```python
from build123d import *

# Parameters (mm, degrees)
F1_DEPTH = 25


with BuildPart() as f1:
    # F0 (on Top) → F1 (new body)
    with BuildSketch(Plane.XY):
        Polygon((0, 40), (-38.992442, 0), (-35.412103, -3.490154), (-12.513641, 20), (0, 32.836992), (13.168698, 20), (37.265833, -3.490154), (41.033594, 0), align=None)
        Polygon((0, 32.836992), (-12.513641, 20), (13.168698, 20), align=None)
    extrude(amount=F1_DEPTH)


solid = f1.part
```
Work out the finished part from the listing and answer in its coordinate system (mm). A direction names the side the tool comes from. Coordinates: 2 decimals unless noted, no trailing zeros. Loops run counter-clockwise (first coordinate to the right, second up) from the corner with the lowest first, then second, coordinate; pieces in that order, holes last.
1) Section B-B (y = 14) is taken. Give the vertices of the cut face in (x, z), plus the area to 3 significant figures.
Results:
outline: (-25.35, 0) - (-18.36, 0) - (-18.36, 25) - (-25.35, 25) - close; (19.32, 0) - (26.67, 0) - (26.67, 25) - (19.32, 25) - close
area: 358 mm2
2) Consider probe 1 along X at (y, z) = (10, 16); probe 2 along X at (y, z) = (7, 10.5); probe 3 along X at (y, z) = (20.5, 15.5). Determine where each line is inside the solid, lowest interval first.
Results:
probe 1: x = -29.24 to -22.26, 23.43 to 30.78
probe 2: x = -32.17 to -25.19, 26.5 to 33.85
probe 3: x = -19.01 to 20
3) Section C-C (x = 6) is taken. Give the vertices of the cut face in (y, z).
Results:
outline: (20, 0) - (34.15, 0) - (34.15, 25) - (20, 25) - close
4) Flat-ended cylindrical pins translate along their axes: pin 1 (8 mm diameter, centred on y = 7.5, z = 5, fed in from +X); pin 2 (3 mm diameter, centred on x = 16.5, z = 3, fed in from +Y); pin 3 (8 mm diameter, centred on x = -26, z = 19.5, fed in from -Y). Find the tip coordinate at first contact, or state that the pin passes through.
Results:
pin 1: stops at x = 37.44
pin 2: stops at y = 25.38
pin 3: stops at y = 2.06
5) Section A-A (z = 14.5) is taken. Give the vertices of the cut face in (x, y), plus the area to 3 significant figures.
Results:
outline: (-38.99, 0) - (-35.41, -3.49) - (-12.51, 20) - (13.17, 20) - (37.27, -3.49) - (41.03, 0) - (0, 40) - close
area: 712 mm2
6) Section D-D (y = 25) is taken. Give the vertices of the cut face in (x, z).
Results:
outline: (-14.62, 0) - (15.39, 0) - (15.39, 25) - (-14.62, 25) - close
7) For faces 1 (the flat face through (-19.223, 20.28, 12.325)), 2 (the flat face through (-24.123, 8.09, 12.325)), determine the directions among +Z, -Z, +X, -X, +Y, -Y from which every point of the face is accessible in a straight line to the end or side of a thin tool.
Results:
face 1: +Z, -Z, -X, +Y
face 2: +Z, -Z, -Y
